```python
from build123d import *

# Parameters (mm, degrees)
SKETCH2_W                     = 5.461
SKETCH2_H                     = 71.755
BOSS_EXTRUDE1_DEPTH           = 3.175
BOSS_EXTRUDE2_DEPTH           = 5.461
CUT_EXTRUDE1_DEPTH            = 2.032
M3_CLEARANCE_HOLE_CLEARENCE_D = 3.3
FILLET1_R                     = 3.175
SKETCH19_R                    = 2
CUT_EXTRUDE2_DEPTH            = 0.500000016
CHAMFER1_SIZE                 = 0.500000016


with BuildPart() as part:
    # Sketch2 → Boss-Extrude1 (new, symmetric)
    with BuildSketch(Plane(origin=(0, 0, 0), x_dir=(1, 0, 0), z_dir=(0, 1, 0))):
        with Locations((0, 12.7)):
            Rectangle(SKETCH2_W, SKETCH2_H)
    extrude(amount=BOSS_EXTRUDE1_DEPTH, both=True)

    # Sketch7 → Boss-Extrude2 (add)
    with BuildSketch(Plane(origin=(-2.7305, 0, 0), x_dir=(0, -1, 0), z_dir=(-1, 0, 0))):
        with BuildLine():
            Line((5.480272256, 15.273700964), (4.627706382, 3.584959425))
            ThreePointArc((4.627706382, 3.584959425), (0, -0.7175), (-4.627706382, 3.584959425))
            Line((-4.627706382, 3.584959425), (-5.480272256, 15.273700964))
            ThreePointArc((-5.480272256, 15.273700964), (0, 24.2625), (5.480272256, 15.273700964))
        make_face()
    extrude(amount=-BOSS_EXTRUDE2_DEPTH)

    # Sketch10 → Cut-Extrude1 (cut)
    with BuildSketch(Plane(origin=(-2.7305, 0, 0), x_dir=(0, -1, 0), z_dir=(-1, 0, 0))):
        with BuildLine():
            Line((-3.114188808, 16.004814628), (-2.221099593, 3.760495073))
            ThreePointArc((-2.221099593, 3.760495073), (0, 1.6955), (2.221099593, 3.760495073))
            Line((2.221099593, 3.760495073), (3.114188808, 16.004814628))
            ThreePointArc((3.114188808, 16.004814628), (0, 21.8495), (-3.114188808, 16.004814628))
        make_face()
    extrude(amount=-CUT_EXTRUDE1_DEPTH, mode=Mode.SUBTRACT)

    # M3 Clearance Hole clearence (through all)
    with Locations(Plane.ZY.offset(2.7305)):
        with Locations((-45.4025, 0)):
            Hole(M3_CLEARANCE_HOLE_CLEARENCE_D / 2)

    # Fillet1
    fillet1_edges = [part.edges().sort_by_distance(p)[0] for p in [
        (0, -3.175, -48.5775),
        (0, 3.175, -48.5775),
    ]]
    fillet(fillet1_edges, radius=FILLET1_R - 0.0001)  # a hair under: the kernel refuses the full size

    # Sketch19 → Cut-Extrude2 (cut)
    with BuildSketch(Plane.ZY.offset(0.6985)):
        with Locations((18.0975, 0)):
            Circle(SKETCH19_R)
    extrude(amount=-CUT_EXTRUDE2_DEPTH, mode=Mode.SUBTRACT)

    # Chamfer1
    chamfer1_edges = [part.edges().sort_by_distance(p)[0] for p in [
        (-0.6985, 0, 16.0975),
    ]]
    chamfer(chamfer1_edges, length=CHAMFER1_SIZE - 0.0001)  # a hair under: the kernel refuses the full size


solid = part.part
```
Verification items for the finished model (mm, model axes). A direction names the side the tool comes from. Round coordinates to 2 decimals unless told otherwise and drop trailing zeros. Order: outer loops, then holes, each group sorted by start corner. A loop starts at its lowest first (then second) coordinate and runs counter-clockwise, first axis right, second up.
1) Material ranges on line 1 (Z direction, x = -2.2, y = 1.25); line 2 (X direction, y = 2.75, z = 16); line 3 (Z direction, x = -0.5, y = -0.5), recorded low to high.
Geometry says:
line 1: z = -48.32 to -46.48, -44.33 to 2.08, 21.64 to 24.13
line 2: x = -0.7 to 2.73
line 3: z = -48.54 to -46.97, -43.83 to 15.85, 20.34 to 24.24
2) Depth check by flat-ended pin: pin 1 (4.5 mm diameter, centred on y = 0, z = 18.1, fed in from -X); pin 2 (1 mm diameter, centred on x = -1.5, z = -25.5, fed in from +Y) (3 decimals); pin 3 (4.5 mm diameter, centred on y = -0.5, z = 18, fed in from -X). Enter the tip coordinate at first touch or a pass-through.
Geometry says:
pin 1: stops at x = -0.45
pin 2: stops at y = 3.175
pin 3: stops at x = -0.7
3) Cross-section at D-D, the plane z = -26. Record the cut outline in (x, y) (1 decimal).
Geometry says:
outline: (-2.7, -3.2) - (2.7, -3.2) - (2.7, 3.2) - (-2.7, 3.2) - close
4) Cross-section at A-A, the plane x = -1.7. Give the number of separate pieces and of enclosed holes in the cut face, plus the area to 3 significant figures.
Geometry says:
separate pieces: 1
enclosed holes: 2
area: 426 mm2
5) Draft check along Y on faces 1 (the cylindrical face through (-0.038, 4.178, 1.903)), 2 (the flat face through (2.73, 0, -4)), 3 (the flat face through (-1.729, 2.674, 9.968)). Enter one of: +Y half, -Y half, draft (parallel to the pull), parting line (faces both ways), or undercut.
Geometry says:
face 1: +Y half
face 2: draft
face 3: undercut
6) Tool access check on faces 4 (the flat face through (0, 3.175, -23)), 5 (the cylindrical face through (0.038, -0.632, -46.927)), 6 (the cylindrical face through (-1.729, -0.114, 21.848)), 7 (the flat face through (0, -3.175, -23)), 8 (the flat face through (-2.73, 0, -12)). Record the directions out of +Z, -Z, +X, -X, +Y, -Y that give a thin tool (end or side, any length) a straight path to the whole face; none if there is none.
Geometry says:
face 4: -Z, +X, -X, +Y
face 5: +X, -X
face 6: -X
face 7: -Z, +X, -X, -Y
face 8: +Z, -Z, -X, +Y, -Y
7) Cross-section at C-C, the plane z = 11.5. Record the cut outline in (x, y), plus the area to 3 significant figures.
Geometry says:
outline: (-2.73, -5.21) - (2.73, -5.21) - (2.73, 5.21) - (-2.73, 5.21) - (-2.73, 2.79) - (-0.7, 2.79) - (-0.7, -2.79) - (-2.73, -2.79) - close
area: 45.5 mm2
